from build123d import *

# Parameters (mm, degrees)
SKETCH1_R            = 3.96875
BOSS_EXTRUDE2_DEPTH  = 40.64
SKETCH4_R            = 1.5875
CUT_EXTRUDE1_DEPTH   = 210.749095026
CUT_EXTRUDE2_START   = 5.08
SKETCH5_R            = 15.875
CUT_EXTRUDE2_DEPTH   = 5.08
SKETCH7_W            = 321.437634852
SKETCH7_H            = 153.081921076
CUT_EXTRUDE3_DEPTH   = 33.02
CUT_EXTRUDE5_DEPTH   = 210.749095026
FILLET1_R            = 6.35
FILLET2_R            = 6.35
EXTRUDE_THIN1_DEPTH  = 10
SKETCH14_R           = 1.950000064
CUT_EXTRUDE6_DEPTH   = 20
BOSS_EXTRUDE4_DEPTH  = 5
MIRROR5_COPY_1_DEPTH = 5
FILLET3_R            = 2.54
SKETCH20_W           = 13.97
SKETCH20_H           = 5.08
BOSS_EXTRUDE5_DEPTH  = 10
FILLET7_SIZE         = 3.81
FILLET7_SIZE_2       = 5.08
FILLET6_SIZE         = 3.81
FILLET6_SIZE_2       = 5.08
CUT_EXTRUDE10_START  = -5
SKETCH19_W           = 7.62
SKETCH19_H           = 10.16
CUT_EXTRUDE10_DEPTH  = 6.27
MIRROR6_OUTLINE_W    = 7.62
MIRROR6_OUTLINE_H    = 5
MIRROR6_DEPTH        = 10
MIRROR6_2_DEPTH      = 10
SKETCH21_W           = 77.087164644
SKETCH21_H           = 69.073945867
CUT_EXTRUDE11_DEPTH  = 210.74909516
SKETCH22_R           = 4.953
BOSS_EXTRUDE6_DEPTH  = 10.16
SKETCH23_R           = 5.08
CUT_EXTRUDE12_DEPTH  = 255.54404949


# Read off the part's stored shape, not the designer's step: Mirror6
with BuildPart() as part:
    # Sketch1 → Boss-Extrude2 (new body)
    with BuildSketch(Plane(origin=(0, 0, 0), x_dir=(1, 0, 0), z_dir=(0, 1, 0))):
        with BuildLine():
            Line((-96.52, 178.942765331), (-55.88, 178.942765331))
            ThreePointArc((-55.88, 178.942765331), (-52.287897552, 177.454867779), (-50.8, 173.862765331))
            Line((-50.8, 173.862765331), (-50.8, 154.610881096))
            ThreePointArc((-50.8, 154.610881096), (-50.750979429, 153.906859803), (-50.604863787, 153.216425724))
            Line((-50.604863787, 153.216425724), (-23.277092285, 57.485544628))
            ThreePointArc((-23.277092285, 57.485544628), (-21.451849938, 54.824742099), (-18.392228498, 53.8))
            Line((-18.392228498, 53.8), (0, 53.8))
            Line((0, 53.8), (0, 0))
            Line((0, 0), (-40.91748188, 0))
            ThreePointArc((-40.91748188, 0), (-43.817717665, 0.909264766), (-45.679732106, 3.31156205))
            Line((-45.679732106, 3.31156205), (-101.282250226, 153.044327381))
            ThreePointArc((-101.282250226, 153.044327381), (-101.519931557, 153.914386555), (-101.6, 154.812765331))
            Line((-101.6, 154.812765331), (-101.6, 173.862765331))
            ThreePointArc((-101.6, 173.862765331), (-100.112102448, 177.454867779), (-96.52, 178.942765331))
        make_face()
        with Locations(Location((-88.9, 166.242765331, 0), (0, 0, 270))):
            Circle(SKETCH1_R, mode=Mode.SUBTRACT)
        with Locations(Location((-63.5, 166.242765331, 0), (0, 0, 270))):
            Circle(SKETCH1_R, mode=Mode.SUBTRACT)
    boss_extrude2 = extrude(amount=BOSS_EXTRUDE2_DEPTH)

    # Mirror1: Boss-Extrude2 across plane
    add(boss_extrude2.mirror(Plane(origin=(0, 40.64, -53.8), x_dir=(0, 0, 1), z_dir=(-1, 0, 0))))

    # Sketch4 → Cut-Extrude1 (cut, through all)
    with BuildSketch(Plane(origin=(0, 40.64, 0), x_dir=(1, 0, 0), z_dir=(0, 1, 0))):
        with Locations(Location((11.548448759, 32.0195, 0), (0, 0, 270))):
            Circle(SKETCH4_R)
        with Locations(Location((0, 12.017, 0), (0, 0, 270))):
            Circle(SKETCH4_R)
        with Locations(Location((-11.548448759, 32.0195, 0), (0, 0, 270))):
            Circle(SKETCH4_R)
    extrude(amount=-CUT_EXTRUDE1_DEPTH, mode=Mode.SUBTRACT)

    # Sketch5 → Cut-Extrude2 (cut)
    with BuildSketch(Plane(origin=(0, 0, 0), x_dir=(1, 0, 0), z_dir=(0, 1, 0)).offset(CUT_EXTRUDE2_START)):
        with Locations(Location((0, 25.352, 0), (0, 0, 270))):
            Circle(SKETCH5_R)
    extrude(amount=CUT_EXTRUDE2_DEPTH, mode=Mode.SUBTRACT)

    # Sketch7 → Cut-Extrude3 (cut)
    with BuildSketch(Plane(origin=(0, 40.64, 0), x_dir=(1, 0, 0), z_dir=(0, 1, 0))):
        with Locations((5.589227859, 76.540960538)):
            Rectangle(SKETCH7_W, SKETCH7_H)
    extrude(amount=-CUT_EXTRUDE3_DEPTH, mode=Mode.SUBTRACT)

    # Sketch8 → Cut-Extrude5 (cut, through all)
    with BuildSketch(Plane(origin=(0, 0, 0), x_dir=(1, 0, 0), z_dir=(0, 1, 0))):
        with BuildLine():
            Line((-3.81, 25.352), (-3.81, 53.8))
            ThreePointArc((-3.81, 53.8), (0, 57.61), (3.81, 53.8))
            Line((3.81, 53.8), (3.81, 25.352))
            ThreePointArc((3.81, 25.352), (0, 21.542), (-3.81, 25.352))
        make_face()
    extrude(amount=CUT_EXTRUDE5_DEPTH, mode=Mode.SUBTRACT)

    # Fillet1
    fillet1_edges = [part.edges().sort_by_distance(p)[0] for p in [
        (-3.81, 3.81, -53.8),
    ]]
    fillet(fillet1_edges, radius=FILLET1_R)

    # Fillet2
    fillet2_edges = [part.edges().sort_by_distance(p)[0] for p in [
        (3.81, 3.81, -53.8),
    ]]
    fillet(fillet2_edges, radius=FILLET2_R)

    # Sketch9 → Extrude-Thin1 (add)
    with BuildSketch(Plane(origin=(0, 0, 0), x_dir=(1, 0, 0), z_dir=(0, 1, 0))):
        Polygon((-91.44, 173.942765331), (-91.44, 224.742765331), (-60.96, 224.742765331), (-60.96, 173.942765331), (-65.96, 173.942765331), (-65.96, 219.742765331), (-86.44, 219.742765331), (-86.44, 173.942765331), align=None)
    extrude_thin1 = extrude(amount=EXTRUDE_THIN1_DEPTH)

    # Sketch14 → Cut-Extrude6 (cut)
    with BuildSketch(Plane.XZ):
        with Locations(Location((-81.2, -174.942765331, 0), (0, 0, 270))):
            Circle(SKETCH14_R)
        with Locations(Location((-71.2, -174.942765331, 0), (0, 0, 270))):
            Circle(SKETCH14_R)
    cut_extrude6 = extrude(amount=-CUT_EXTRUDE6_DEPTH, mode=Mode.SUBTRACT)

    # Sketch18 → Boss-Extrude4 (add)
    with BuildSketch(Plane(origin=(-60.96, 10, -178.942765331), x_dir=(0, 0, 1), z_dir=(-1, 0, 0))):
        Polygon((-1.27, 0), (0, 1.524), (0, 0), align=None)
    boss_extrude4 = extrude(amount=BOSS_EXTRUDE4_DEPTH)

    # Mirror3: Boss-Extrude4 across plane
    add(boss_extrude4.mirror(Plane(origin=(-76.2, 0, 0), x_dir=(0, 0, 1), z_dir=(1, 0, 0))))

    # Mirror5: Extrude-Thin1, Cut-Extrude6, Boss-Extrude4 across plane
    add(extrude_thin1.mirror(Plane(origin=(0, 0, 0), x_dir=(0, 0, 1), z_dir=(1, 0, 0))))
    add(cut_extrude6.mirror(Plane(origin=(0, 0, 0), x_dir=(0, 0, 1), z_dir=(1, 0, 0))), mode=Mode.SUBTRACT)
    add(boss_extrude4.mirror(Plane(origin=(0, 0, 0), x_dir=(0, 0, 1), z_dir=(1, 0, 0))))

    # Mirror5 copy 1 sketch → Mirror5 copy 1 (add)
    with BuildSketch(Plane(origin=(91.44, 10, -178.942765331), x_dir=(0, 0, 1), z_dir=(-1, 0, 0))):
        Polygon((-1.27, 0), (0, 1.524), (0, 0), align=None)
    extrude(amount=MIRROR5_COPY_1_DEPTH)

    # Fillet3
    fillet3_edges = [part.edges().sort_by_distance(p)[0] for p in [
        (-91.44, 5, -224.742765331),
        (-60.96, 5, -224.742765331),
        (91.44, 5, -224.742765331),
        (60.96, 5, -224.742765331),
    ]]
    fillet(fillet3_edges, radius=FILLET3_R)

    # Sketch20 → Boss-Extrude5 (add)
    with BuildSketch(Plane(origin=(0, 0, 0), x_dir=(1, 0, 0), z_dir=(0, 1, 0))):
        with Locations((-76.2, 227.282765331)):
            Rectangle(SKETCH20_W, SKETCH20_H)
    extrude(amount=BOSS_EXTRUDE5_DEPTH)

    # Fillet7
    # an asymmetric fillet: 5.08, 3.81 mm, written as the material it takes off along each edge
    with BuildSketch(Plane(origin=(-83.185, -12.7, -229.822765331), x_dir=(0, 0, 1), z_dir=(0, 1, 0))) as fillet7_piece_1:
        with BuildLine():
            Bezier((FILLET7_SIZE, 0), (0, 0), (0, FILLET7_SIZE_2), weights=[1, 0.707106781, 1])
            Line((0, FILLET7_SIZE_2), (0, 0))
            Line((0, 0), (FILLET7_SIZE, 0))
        make_face()
    extrude(amount=35.4, mode=Mode.SUBTRACT)

    # Fillet6
    # an asymmetric fillet: 5.08, 3.81 mm, written as the material it takes off along each edge
    with BuildSketch(Plane(origin=(-69.215, -12.7, -229.822765331), x_dir=(0, 0, 1), z_dir=(0, 1, 0))) as fillet6_piece_1:
        with BuildLine():
            Bezier((FILLET6_SIZE, 0), (0, 0), (0, -FILLET6_SIZE_2), weights=[1, 0.707106781, 1])
            Line((0, -FILLET6_SIZE_2), (0, 0))
            Line((0, 0), (FILLET6_SIZE, 0))
        make_face()
    extrude(amount=35.4, mode=Mode.SUBTRACT)

    # Sketch19 → Cut-Extrude10 (cut)
    with BuildSketch(Plane(origin=(0, 0, -224.742765331), x_dir=(-1, 0, 0), z_dir=(0, 0, -1)).offset(CUT_EXTRUDE10_START)):
        with Locations((76.2, 4.92)):
            Rectangle(SKETCH19_W, SKETCH19_H)
    extrude(amount=CUT_EXTRUDE10_DEPTH, mode=Mode.SUBTRACT)

    # Mirror6 outline → Mirror6 (cut)
    with BuildSketch(Plane(origin=(0, 0, 0), x_dir=(1, 0, 0), z_dir=(0, 1, 0))):
        with Locations((76.2, 222.242765331)):
            Rectangle(MIRROR6_OUTLINE_W, MIRROR6_OUTLINE_H)
    extrude(amount=MIRROR6_DEPTH, mode=Mode.SUBTRACT)

    # Mirror6 2 outline → Mirror6 2 (add)
    with BuildSketch(Plane(origin=(0, 0, 0), x_dir=(1, 0, 0), z_dir=(0, 1, 0))):
        with BuildLine():
            add(Edge.make_bspline(
                [(78.105, 229.822765331), (83.185, 229.822765331), (83.185, 226.012765331)],
                knots=[0, 0, 0, 1, 1, 1], degree=2, weights=[1, 0.707106781, 1]))
            Line((78.105, 229.822765331), (74.295, 229.822765331))
            add(Edge.make_bspline(
                [(69.215, 226.012765331), (69.215, 229.822765331), (74.295, 229.822765331)],
                knots=[0, 0, 0, 1, 1, 1], degree=2, weights=[1, 0.707106781, 1]))
            Line((69.215, 226.012765331), (69.215, 224.742765331))
            Line((69.215, 224.742765331), (72.39, 224.742765331))
            Line((72.39, 224.742765331), (72.39, 226.012765331))
            Line((72.39, 226.012765331), (80.01, 226.012765331))
            Line((80.01, 226.012765331), (80.01, 224.742765331))
            Line((80.01, 224.742765331), (83.185, 224.742765331))
            Line((83.185, 224.742765331), (83.185, 226.012765331))
        make_face()
    extrude(amount=MIRROR6_2_DEPTH)

    # Sketch21 → Cut-Extrude11 (cut, through all)
    with BuildSketch(Plane(origin=(0, 0, -178.942765331), x_dir=(-1, 0, 0), z_dir=(0, 0, -1))):
        with Locations((78.752430528, 22.788762469)):
            Rectangle(SKETCH21_W, SKETCH21_H)
    extrude(amount=CUT_EXTRUDE11_DEPTH, mode=Mode.SUBTRACT)

    # Sketch22 → Boss-Extrude6 (add)
    with BuildSketch(Plane.XZ):
        with Locations(Location((-60.96, -109.572454465, 0), (0, 0, 90))):
            Circle(SKETCH22_R)
    extrude(amount=BOSS_EXTRUDE6_DEPTH)

    # Sketch23 → Cut-Extrude12 (cut, through all)
    with BuildSketch(Plane.XZ):
        with Locations((-67.31, -98.573931837)):
            Circle(SKETCH23_R)
        with Locations((-71.958522628, -103.222454465)):
            Circle(SKETCH23_R)
        with Locations((-60.96, -96.872454465)):
            Circle(SKETCH23_R)
        with Locations((-54.61, -98.573931837)):
            Circle(SKETCH23_R)
        with Locations((-49.961477372, -103.222454465)):
            Circle(SKETCH23_R)
    extrude(amount=-CUT_EXTRUDE12_DEPTH, mode=Mode.SUBTRACT)


solid = part.part
Can you work these out from the model? Positions are in its coordinate system, mm. A direction names the side the tool comes from. Coordinates: 2 decimals unless noted, no trailing zeros. Write each loop counter-clockwise with the first axis right and the second up, starting at its lowest first coordinate (ties: lowest second). Pieces come first, ordered by that corner, then holes. Notation, with made-up numbers: (-9.75, -35) - (-2.75, -35) arc R11 ccw to (-2.75, -14) - close; hole circle Ø5 at (82, 38). An arc over 180 degrees is marked (long way). Return JSON: item names as keys, results as strings. Group by question number.
Item 1: If we section it at B-B (z = -212): Write out the boundary of the cut face in (x, y).
Item 2: We'd pull the mould along Z, two halves only. Please class faces 4 (the face through (43.782, 3.757, -0.885)), 5 (the face through (76, 40.64, -166)), 6 (the face through (76, 5, -226.013)): pulls with the +Z half, pulls with the -Z half, needs draft (parallel to the pull), parting line crosses it, or undercut.
Item 3: If we section it at C-C (z = -18.5): Write out the boundary of the cut face in (x, y), then the cut area to 3 significant figures.
Item 4: Which directions (+Z, -Z, +X, -X, +Y, -Y) give clear straight access to the entire face, cutting with the end or side of a thin tool? Please do faces 1 (the face through (5.62, 3.86, -51.89)), 2 (the face through (83, 5, -219.743)), 3 (the face through (87, 10, -205)).
Item 5: If we section it at A-A (y = 32.5): Write out the boundary of the cut face in (x, z), then the cut area to 3 significant figures.
Item 6: If we section it at D-D (x = 28.5): Write out the boundary of the cut face in (y, z).
Item 7: Please list where these lines run through material, in increasing order: probe 1 along Y at (x, z) = (90, -193); probe 2 along Z at (x, y) = (-81, 15); probe 3 along Y at (x, z) = (47.5, -134).
Item 8: I'm going to push flat-ended pins straight in: pin 1 Ø3 at (y, z) = (7, -222) entering from -X; pin 2 Ø2 at (x, z) = (-63.5, -136) entering from +Y; pin 3 Ø1.2 at (x, z) = (-82, -175.5) entering from -Y. Where does each tip first touch, or does it pass through?
Return value:
{
 "1": {"outline": "(60.96, 0) - (65.96, 0) - (65.96, 10) - (60.96, 10) - close; (86.44, 0) - (91.44, 0) - (91.44, 10) - (86.44, 10) - close"},
 "2": {"face 4": "pulls with the +Z half", "face 5": "needs draft", "face 6": "undercut"},
 "3": {"outline": "(-51.32, 0) - (51.32, 0) - (51.32, 7.62) - (14.32, 7.62) - (14.32, 5.08) - (-14.32, 5.08) - (-14.32, 7.62) - (-51.32, 7.62) - close", "area": "709 mm^2"},
 "4": {"face 1": "-Z, +Y, -Y", "face 2": "+Y, -Y", "face 3": "-Z, +X, -X, +Y"},
 "5": {"outline": "(-101.6, -173.86) arc R5.08 ccw to (-96.52, -178.94) - (-55.88, -178.94) arc R5.08 ccw to (-50.8, -173.86) - (-50.8, -154.61) arc R5.08 cw to (-50.6, -153.22) - (-50.57, -153.08) - (-101.3, -153.08) arc R5.08 ccw to (-101.6, -154.81) - close; (50.57, -153.08) - (50.6, -153.22) arc R5.08 cw to (50.8, -154.61) - (50.8, -173.86) arc R5.08 ccw to (55.88, -178.94) - (96.52, -178.94) arc R5.08 ccw to (101.6, -173.86) - (101.6, -154.81) arc R5.08 ccw to (101.3, -153.08) - close; hole circle Ø7.94 at (-88.9, -166.24); hole circle Ø7.94 at (-63.5, -166.24); hole circle Ø7.94 at (63.5, -166.24); hole circle Ø7.94 at (88.9, -166.24)", "area": "2,410 mm^2"},
 "6": {"outline": "(0, -75.78) - (7.62, -75.78) - (7.62, 0) - (0, 0) - close"},
 "7": {"probe 1": "y = 0 to 10", "probe 2": "z = -178.94 to -176.88, -173 to -153.08", "probe 3": "y = 0 to 7.62"},
 "8": {"pin 1": "stops at x = 60.96", "pin 2": "stops at y = 7.62", "pin 3": "stops at y = 20"}
}
